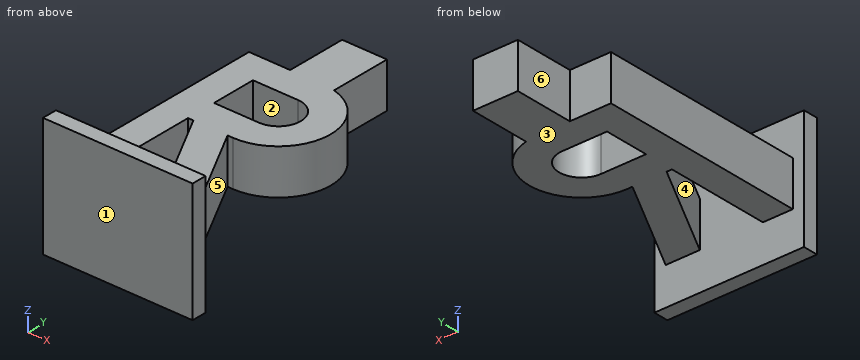
from build123d import *

# Parameters (mm, degrees)
AUFSATZ_LINEAR_AUSTRAGEN1_DEPTH = 15
SKIZZE2_W                       = 50
SKIZZE2_H                       = 40
AUFSATZ_LINEAR_AUSTRAGEN2_DEPTH = 5
SKIZZE6_W                       = 15
SKIZZE6_H                       = 20.406507086
AUFSATZ_LINEAR_AUSTRAGEN3_DEPTH = 15


with BuildPart() as part:
    # Skizze1 → Aufsatz-Linear austragen1 (new body)
    with BuildSketch(Plane.XY):
        with BuildLine():
            Line((0, 0), (0, 70))
            Line((0, 70), (25, 70))
            ThreePointArc((25, 70), (42.5, 52.5), (25, 35))
            Line((25, 35), (23.209169398, 35))
            Line((23.209169398, 35), (42.5, 0))
            Line((42.5, 0), (31.081661205, 0))
            Line((31.081661205, 0), (11.790830602, 35))
            Line((11.790830602, 35), (10, 35))
            Line((10, 35), (10, 0))
            Line((10, 0), (0, 0))
        make_face()
        with BuildLine():
            Line((10, 60), (10, 45))
            Line((10, 45), (25, 45))
            ThreePointArc((25, 45), (32.5, 52.5), (25, 60))
            Line((25, 60), (10, 60))
        make_face(mode=Mode.SUBTRACT)
    extrude(amount=AUFSATZ_LINEAR_AUSTRAGEN1_DEPTH)

    # Skizze2 → Aufsatz-Linear austragen2 (add)
    with BuildSketch(Plane.XZ):
        with Locations((21.25, 7.5)):
            Rectangle(SKIZZE2_W, SKIZZE2_H)
    extrude(amount=AUFSATZ_LINEAR_AUSTRAGEN2_DEPTH)

    # Skizze6 → Aufsatz-Linear austragen3 (add)
    with BuildSketch(Plane.XY.offset(15)):
        with Locations((21.25, 79.796746457)):
            Rectangle(SKIZZE6_W, SKIZZE6_H)
    extrude(amount=-AUFSATZ_LINEAR_AUSTRAGEN3_DEPTH)


solid = part.part
Input: part model. Units: mm. Frame: model coordinates. Face numbers are marked on the shaded views. A direction names the side the tool comes from. Round coordinates to 2 decimals unless told otherwise and drop trailing zeros. Order: outer loops, then holes, each group sorted by start corner. A loop starts at its lowest first (then second) coordinate and runs counter-clockwise, first axis right, second up.
1. Cut plane D-D, the plane x = 34. Output: boundary loops of the cut face in (y, z), then the cut area to 3 significant figures.
The answers:
outline: (-5, -12.5) - (0, -12.5) - (0, 0) - (15.42, 0) - (15.42, 15) - (0, 15) - (0, 27.5) - (-5, 27.5) - close; (37.49, 0) - (67.51, 0) - (67.51, 15) - (37.49, 15) - close
area: 882 mm2
2. Cut plane C-C, the plane x = 21. Output: boundary loops of the cut face in (y, z).
The answers:
outline: (-5, -12.5) - (0, -12.5) - (0, 27.5) - (-5, 27.5) - close; (18.29, 0) - (45, 0) - (45, 15) - (18.29, 15) - close; (60, 0) - (90, 0) - (90, 15) - (60, 15) - close
3. Mould query, pull axis Y, two halves, no side actions, for the marked faces 1, 2 and 3. Classes: released by +Y, released by -Y, zero draft, split by the parting line, or undercut.
The answers:
face 1: released by -Y
face 2: undercut
face 3: zero draft
4. Cut plane B-B, the plane x = 5.5. Output: boundary loops of the cut face in (y, z).
The answers:
outline: (-5, -12.5) - (0, -12.5) - (0, 0) - (70, 0) - (70, 15) - (0, 15) - (0, 27.5) - (-5, 27.5) - close
5. Set-up query: the marked faces 4, 5 and 6. Return all of +Z, -Z, +X, -X, +Y, -Y with unobstructed straight access to the full face (end or side cutting, diameter ignored); none if empty.
The answers:
face 4: +Z, -Z
face 5: +Z, -Z, +X
face 6: +Z, -Z, -X, +Y
6. Cut plane A-A, the plane y = 52.5. Output: boundary loops of the cut face in (x, z), then the cut area to 3 significant figures.
The answers:
outline: (0, 0) - (10, 0) - (10, 15) - (0, 15) - close; (32.5, 0) - (42.5, 0) - (42.5, 15) - (32.5, 15) - close
area: 300 mm2
7. Pin query (flat end, axial travel): P1, Ø5, axis at x = 25, y = 67.5, coming from the +Z side; P2, Ø2, axis at y = 57.5, z = -0.5, coming from the +X side; P3, Ø1.5, axis at x = 20, z = -3, coming from the +Y side; P4, Ø5, axis at y = 11.5, z = -4, coming from the +X side. Return the tip coordinate at first contact, or that it passes through.
The answers:
P1: stops at z = 15
P2: stops at x = 42
P3: stops at y = 0
P4: passes through
8. Material intervals for line 1 (Y direction, x = 25.5, z = 14.5); line 2 (Y direction, x = 38, z = 25); line 3 (Y direction, x = 24, z = 5), sorted ascending.
The answers:
line 1: y = -5 to 0, 10.13 to 30.84, 35.01 to 45.02, 59.98 to 90
line 2: y = -5 to 0
line 3: y = -5 to 0, 12.85 to 33.57, 35 to 45, 60 to 90
